Verification items for the finished model (mm, model axes). Coordinates: 2 decimals unless noted, no trailing zeros. Write each loop counter-clockwise with the first axis right and the second up, starting at its lowest first coordinate (ties: lowest second). Pieces come first, ordered by that corner, then holes. Notation, with made-up numbers: (10, -30.5) -> (26, -30.5) arc R24 ccw to (26, -13.5) -> close; hole circle Ø6 at (51, 27). An arc over 180 degrees is marked (long way). Answer in a Markdown table with one row per item.
Autodesk Inventor part; units mm, degrees
ref_plane "Start plane" through (0, 0, -18.7744) normal (0, 0, 1) x (1, 0, 0)
ref_plane "End plane" through (0, 0, 368.7744) normal (0, 0, 1) x (1, 0, 0)
ref_plane "Work Plane4" through (16.6257, 2.1487, 366.764) normal (-0.7013, -0.0906, 0.7071) x (0.7119, -0.0372, 0.7013)
ref_plane "Start plane" through (0, 0, -18.7744) normal (0, 0, 1) x (1, 0, 0)
ref_plane "End plane" through (0, 0, 368.7744) normal (0, 0, 1) x (1, 0, 0)
sketch "Sketch" plane through (0, 0, 0) normal (0, 0, 1) x (1, 0, 0)
  circle A0 centre (0, 0) radius 13.3858
  circle A1 centre (0, 0) radius 16.764
  dimension "d0" = 33.528
  dimension "d1" = 3.3782
extrude "Body" add sketch "Sketch" along normal up to surface (387.5489 mm away) from surface at -18.7744
sketch "Sketch3" plane through (0, 0, 0) normal (0, 0, 1) x (1, 0, 0)
  line L0 (0, 0) -> (10, 0)
ref_plane "Work Plane3" through (0, 0, 0) normal (0, -1, 0) x (1, 0, 0)
ref_plane "Work Plane4" through (16.6257, 2.1487, 366.764) normal (-0.7013, -0.0906, 0.7071) x (0.7119, -0.0372, 0.7013)
split "Split1" plane through (16.6257, 2.1487, 366.764) removes the side toward (-0.7013, -0.0906, 0.7071)
ref_plane "Work Plane5" through (16.6257, 2.1487, -16.764) normal (-0.7013, -0.0906, -0.7071) x (-0.6791, -0.217, 0.7013)
split "Split2" plane through (16.6257, 2.1487, -16.764) removes the side toward (-0.7013, -0.0906, -0.7071)
sketch "Sketch4" plane through (0, 0, 0) normal (0, -1, 0) x (1, 0, 0)
  line L0 (-2, -18.7744) -> (12, -18.7744)
  line L1 (-2, 368.7744) -> (12, 368.7744)
  dimension "d7" = 387.5489
equation "\"d0\" = G_H"
equation "\"d1\" = G_T"
equation "\"d2\" = G_L"
equation "\"G_H\" = 33.528"
equation "\"G_T\" = 3.3782"
equation "\"G_L\" = 383.528"
equation "\"G_OFFSET_START\" = 18.77444"
equation "\"G_OFFSET_END\" = 18.77444"
equation "\"d4\" = -G_OFFSET_START"
equation "\"d5\" = G_OFFSET_END + B_L"
equation "\"B_L\" = 350"
properties part number "ANSI - 1 x 0.133 - 15.1" material "Steel, Mild"
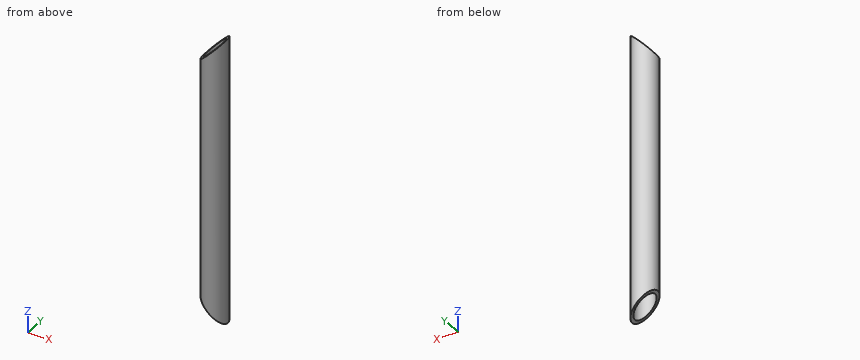
1. Sectioned sample at A-A, the plane y = -9.5. Record the cut outline in (x, z).
Findings below:
| item | result |
|---|---|
| outline | (-13.81, 14.92) -> (-9.43, 10.57) -> (-9.43, 339.43) -> (-13.81, 335.08) -> close; (9.43, -8.14) -> (13.81, -12.48) -> (13.81, 362.48) -> (9.43, 358.14) -> close |
2. Material ranges on probe 1 along Y at (x, z) = (0, 75); probe 2 along Y at (x, z) = (5.5, 99), recorded low to high. Write a range as from..to.
Findings below:
| item | result |
|---|---|
| probe 1 | y = -16.76..-13.39, 13.39..16.76 |
| probe 2 | y = -15.84..-12.2, 12.2..15.84 |
3. Sectioned sample at C-C, the plane z = 205. Record the cut outline in (x, y).
Findings below:
| item | result |
|---|---|
| outline | circle Ø33.53 at (0, 0); hole circle Ø26.77 at (0, 0) |
4. Go/stop test with flat-tipped pins: pin 1 (1.5 mm diameter, centred on y = 11.5, z = 187, fed in from -X); pin 2 (3 mm diameter, centred on x = 9, z = 72, fed in from +Y); pin 3 (4 mm diameter, centred on x = 8, z = 25, fed in from +Y). Record where each tip stops, or that it passes through.
Findings below:
| item | result |
|---|---|
| pin 1 | stops at x = -12.86 |
| pin 2 | stops at y = 14.99 |
| pin 3 | stops at y = 15.65 |
5. Sectioned sample at B-B, the plane x = -5. Record the cut outline in (y, z).
Findings below:
| item | result |
|---|---|
| outline | (-16, 7.01) -> (-12.42, 6.55) -> (-12.42, 343.45) -> (-16, 342.99) -> close; (12.42, 3.37) -> (16, 2.91) -> (16, 347.09) -> (12.42, 346.63) -> close |
